Part model, mm, in its own coordinate system. A direction names the side the tool comes from. Give positions to 0.01 mm unless a question says otherwise; leave off trailing zeros. Write each loop counter-clockwise with the first axis right and the second up, starting at its lowest first coordinate (ties: lowest second). Pieces come first, ordered by that corner, then holes. Notation, with made-up numbers: M 15,-18.75 L 58,-18.75 A24 ccw 58,4.25 Z; hole C -8.5,63.25 d2. An arc over 180 degrees is marked long. Answer as CSV lines item,"result". Start each with the question number.
1) Tool access for faces 4 (the cylindrical face through (-29, 5, 28)), 5 (the cylindrical face through (-25, 6, 4)): list every direction of +Z, -Z, +X, -X, +Y, -Y with a clear straight run to the whole face (end or side of a thin tool).
2) Wall check: line 1 along Z through (x, y) = (-20.5, 9.25); line 2 along X through (y, z) = (9, 17.5); line 3 along Y through (x, z) = (-16.25, 22.75). Give the ranges that are in metal, low to high. Write a range as from..to.
3) Slice it at B-B, the plane y = 3.5. Give the cut face in (x, z).
4) Slice it at A-A, the plane x = -10. Give the cut face in (y, z), plus the area to 3 significant figures.
5) Pin check, flat tips, straight feed: pin 1 Ø1.5 at (y, z) = (4.5, 26) entering from +X; pin 2 Ø7 at (x, z) = (-15.5, 21) entering from +Y. Stop position of each tip, or through.
6) Mould opens along X. For faces 1 (the flat face through (-15, 6, 3)), 2 (the cylindrical face through (-2, 5, 29)), 3 (the flat face through (-15, 0, 15)) say: pulls with the +X half, pulls with the -X half, needs draft (parallel to the pull), parting line crosses it, or undercut.
7) Slice it at C-C, the plane z = 16.75. Give the cut face in (x, y), plus the area to 3 significant figures.
```python
from build123d import *

# Parameters (mm, degrees)
SKETCH2_W           = 30
SKETCH2_H           = 30
BOSS_EXTRUDE1_DEPTH = 10
SKETCH4_W           = 24
SKETCH4_H           = 24
CUT_EXTRUDE1_DEPTH  = 8
FILLET1_R           = 5
FILLET2_R           = 5


with BuildPart() as part:
    # Sketch2 → Boss-Extrude1 (new body)
    with BuildSketch(Plane(origin=(0, 0, 0), x_dir=(1, 0, 0), z_dir=(0, 1, 0))):
        with Locations((-15, -15)):
            Rectangle(SKETCH2_W, SKETCH2_H)
    extrude(amount=BOSS_EXTRUDE1_DEPTH)

    # Sketch4 → Cut-Extrude1 (cut)
    with BuildSketch(Plane(origin=(0, 10, 0), x_dir=(1, 0, 0), z_dir=(0, 1, 0))):
        with Locations((-15, -15)):
            Rectangle(SKETCH4_W, SKETCH4_H)
    extrude(amount=-CUT_EXTRUDE1_DEPTH, mode=Mode.SUBTRACT)

    # Fillet1
    fillet1_edges = [part.edges().sort_by_distance(p)[0] for p in [
        (0, 5, 30),
        (-30, 5, 30),
        (-30, 5, 0),
        (0, 5, 0),
    ]]
    fillet(fillet1_edges, radius=FILLET1_R)

    # Fillet2
    fillet2_edges = [part.edges().sort_by_distance(p)[0] for p in [
        (-27, 6, 27),
        (-27, 6, 3),
        (-3, 6, 3),
        (-3, 6, 27),
    ]]
    fillet(fillet2_edges, radius=FILLET2_R)


solid = part.part
```
Found:
1,face 4,"+Z, -X, +Y, -Y"
1,face 5,"+Y"
2,line 1,"0..3, 27..30"
2,line 2,"-30..-27, -3..0"
2,line 3,"0..2"
3,outline,"M -30,5 A5 ccw -25,0 L -5,0 A5 ccw 0,5 L 0,25 A5 ccw -5,30 L -25,30 A5 ccw -30,25 Z; hole M -27,8 A5 ccw -22,3 L -8,3 A5 ccw -3,8 L -3,22 A5 ccw -8,27 L -22,27 A5 ccw -27,22 Z"
4,outline,"M 0,0 L 10,0 L 10,3 L 2,3 L 2,27 L 10,27 L 10,30 L 0,30 Z"
4,area,"108 mm²"
5,pin 1,"x = -0.01"
5,pin 2,"y = 2"
6,face 1,"undercut"
6,face 2,"pulls with the +X half"
6,face 3,"needs draft"
7,outline,"M -30,0 L 0,0 L 0,10 L -3,10 L -3,2 L -27,2 L -27,10 L -30,10 Z"
7,area,"108 mm²"
